Autodesk Inventor part; units mm, degrees
ref_plane "YZ Plane" through (0, 0, 0) normal (1, 0, 0) x (0, 1, 0)
ref_plane "XZ Plane" through (0, 0, 0) normal (0, 1, 0) x (-1, 0, 0)
ref_plane "XY Plane" through (0, 0, 0) normal (0, 0, 1) x (1, 0, 0)
sketch "Skizze1" plane through (0, 0, 0) normal (0, 1, 0) x (-1, 0, 0)
  line L0 (-25, 30) -> (25, 30)
  line L1 (25, 30) -> (25, -30)
  line L2 (25, -30) -> (-25, -30)
  line L3 (-25, -30) -> (-25, 30)
  line L4 (-25, 30) -> (25, -30) construction
  line L5 (25, 30) -> (-25, -30) construction
  point P0 (0, 0)
  dimension "d0" = 50
  dimension "d1" = 60
extrude "Extrusion1" add sketch "Skizze1" along normal blind 5
sketch "Skizze2" plane through (0, 5, 0) normal (0, 1, 0) x (1, 0, 0)
  line L0 (-25, -30) -> (25, -30)
  line L1 (25, -30) -> (25, 30)
  line L2 (25, 30) -> (-25, 30)
  line L3 (-25, 30) -> (-25, -30)
  line L4 (25, -30) -> (25, 30)
  line L5 (25, 30) -> (20, 30)
  line L6 (20, 30) -> (20, -12)
  line L7 (20, -12) -> (25, -12)
  line L8 (25, -12) -> (25, 30)
  point P0 (0, 0)
  dimension "d8" = 5
  dimension "d9" = 42
extrude "Extrusion2" add sketch "Skizze2" along normal blind 38 contours L7 L6 L2 L1
sketch "Skizze3" plane through (25, 0, 30) normal (1, 0, 0) x (0, 0, -1)
  line L0 (60, 0) -> (0, 0)
  line L1 (60, 0) -> (60, 43)
  line L2 (18, 43) -> (60, 43)
  line L3 (18, 5) -> (18, 43)
  line L4 (0, 5) -> (18, 5)
  line L5 (0, 0) -> (0, 5)
  line L6 (39, -5.2039) -> (39, 72.0028) construction
  line L7 (23.5, 6.5) -> (54.5, 6.5) construction
  line L8 (54.5, 6.5) -> (54.5, 37.5) construction
  line L9 (54.5, 37.5) -> (23.5, 37.5) construction
  line L10 (23.5, 37.5) -> (23.5, 6.5) construction
  line L11 (23.5, 6.5) -> (54.5, 37.5) construction
  line L12 (54.5, 6.5) -> (23.5, 37.5) construction
  point P0 (30, 0)
  point P1 (39, 22)
  dimension "d10" = 21
  dimension "d11" = 17
  dimension "d19" = 31
  dimension "d20" = 31
hole "Bohrung1" at (25, 22, -9) direction (-1, 0, 0) diameter 24 end through all
hole "Bohrung2" at (25, 37.5, 6.5) at (25, 37.5, -24.5) direction (-1, 0, 0) diameter 4 end through all
sketch "Skizze5" plane through (0, 0, 0) normal (0, -1, 0) x (1, 0, 0)
  line L0 (25, 30) -> (-25, 30)
  line L1 (-25, 30) -> (-25, -30)
  line L2 (-25, -30) -> (25, -30)
  line L3 (25, -30) -> (25, 30)
  line L4 (32.3204, 18.7) -> (-38.6965, 18.7) construction
  point P0 (0, 0)
  point P1 (-15, 18.7)
  point P2 (5, 18.7)
  dimension "d31" = 11.3
  dimension "d32" = 10
  dimension "d33" = 20
hole "Bohrung3" at (-15, 0, 18.7) at (5, 0, 18.7) direction (0, 1, 0) diameter 4 end through all counterbore diameter 8 counterbore depth 3
properties part number "Backplate"
Geometry check sheet. Reference: the model listing, model coordinates, mm. A direction names the side the tool comes from. Give positions to 0.01 mm unless a question says otherwise; leave off trailing zeros. Loops run counter-clockwise (first coordinate to the right, second up) from the corner with the lowest first, then second, coordinate; pieces in that order, holes last. Notation, with made-up numbers: M 30,69.25 L 59,69.25 A22 ccw 59,90.25 Z; hole C 14.5,20.25 d3. An arc over 180 degrees is marked long. Write item = value, one per line.
(1) Sectioned sample at D-D, the plane z = -24.5. Record the cut outline in (x, y).
Answer below:
outline = M -25,0 L 25,0 L 25,35.5 L 20,35.5 L 20,5 L -25,5 Z; M 20,39.5 L 25,39.5 L 25,43 L 20,43 Z
(2) Material ranges on line 1 (X direction, y = 2.25, z = 18.7); line 2 (Z direction, x = 23.1, y = 37.5); line 3 (Z direction, x = 5, y = 2.2), recorded low to high. Write a range as [from, to].
Answer below:
line_1 = [-25, -19], [-11, 1], [9, 25]
line_2 = [-30, -26.5], [-22.5, 4.5], [8.5, 12]
line_3 = [-30, 14.7], [22.7, 30]
(3) Sectioned sample at C-C, the plane y = 33. Record the cut outline in (x, z).
Answer below:
outline = M 20,-30 L 25,-30 L 25,-13.8 L 20,-13.8 Z; M 20,-4.2 L 25,-4.2 L 25,12 L 20,12 Z
(4) Release check for a two-part mould opening along Z. For faces 1 (the face through (22, 24, 12)), 2 (the face through (0, 0, 0)), 3 (the face through (6, 3, 21)), 4 (the face through (6.532, 1.521, 15.005)) record: released by +Z, released by -Z, zero draft, split by the parting line, or undercut.
Answer below:
face_1 = released by +Z
face_2 = zero draft
face_3 = undercut
face_4 = undercut
(5) Tool access check on faces 5 (the face through (22, 43, -9)), 6 (the face through (20, 32, 0)), 7 (the face through (-14, 3, 21)). Record the directions out of +Z, -Z, +X, -X, +Y, -Y that give a thin tool (end or side, any length) a straight path to the whole face; none if there is none.
Answer below:
face_5 = +Z, -Z, +X, -X, +Y
face_6 = +Z, -Z, -X, +Y
face_7 = -Y
(6) Gauge pin test, flat ends, axial feed: pin 1 Ø4.5 at (y, z) = (37.5, 6.5) entering from -X; pin 2 Ø1.5 at (x, y) = (22.5, 29) entering from +Z. Record the tip position at first contact, or that the pin passes through.
Answer below:
pin_1 = 20
pin_2 = 12
(7) Sectioned sample at B-B, the plane x = -15. Record the cut outline in (y, z).
Answer below:
outline = M 0,-30 L 5,-30 L 5,16.7 L 3,16.7 L 3,14.7 L 0,14.7 Z; M 0,22.7 L 3,22.7 L 3,20.7 L 5,20.7 L 5,30 L 0,30 Z
(8) Sectioned sample at A-A, the plane z = -9. Record the cut outline in (x, y), plus the area to 3 significant figures.
Answer below:
outline = M -25,0 L 25,0 L 25,10 L 20,10 L 20,5 L -25,5 Z; M 20,34 L 25,34 L 25,43 L 20,43 Z
area = 320 mm2
